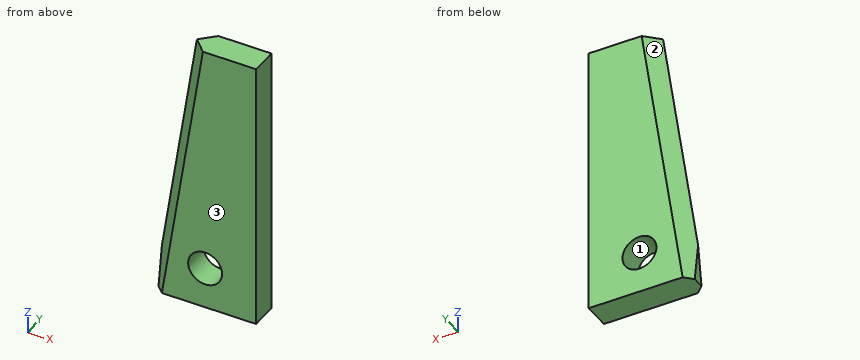
from build123d import *

# Parameters (mm, degrees)
F0_W     = 19.05
F0_H     = 50.8
F1_DEPTH = 5.08
F3_D     = 6.35
F5_DEPTH = 25.4
F6_SIZE  = 2.53999


# Not quite as in the source:
# - a fillet or chamfer is up to 0.001 mm smaller than in the source, because OpenCascade refuses the exact size


with BuildPart() as f1:
    # F0 (on Front) → F1 (new body)
    with BuildSketch(Plane.XZ):
        with Locations((-9.525, 25.4)):
            Rectangle(F0_W, F0_H)
    extrude(amount=F1_DEPTH)

    # F3 (through all)
    with Locations(Plane.XZ.offset(5.08)):
        with Locations((-9.525, 7.7354544774)):
            Hole(F3_D / 2)

    # F4 (on face) → F5 (cut)
    with BuildSketch(Plane.XZ.offset(5.08)):
        Polygon((-19.05, 7.4566449039), (-12.5023688375, 50.8), (-19.05, 50.8), align=None)
    extrude(amount=-F5_DEPTH, mode=Mode.SUBTRACT)

    # F6 (size 2.54 in the source; OpenCascade refuses exactly that, so slightly less here)
    f6_edges = [f1.edges().sort_by_distance(p)[0] for p in [
        (-15.776184, -5.08, 29.128322),
        (-15.776184, 0, 29.128322),
    ]]
    chamfer(f6_edges, length=F6_SIZE)


solid = f1.part
Read the model definition and answer for the solid it produces. Units are mm, in the model's axes. Face numbers are marked on the shaded views. Round coordinates to 2 decimals unless told otherwise and drop trailing zeros. Order: outer loops, then holes, each group sorted by start corner. A loop starts at its lowest first (then second) coordinate and runs counter-clockwise, first axis right, second up. Notation, with made-up numbers: (42, 56.25) - (99, 56.25) arc R21 cw to (99, 82.25) - close; hole circle Ø2 at (-10.5, -33). An arc over 180 degrees is marked (long way). Use one line per item in the form item = value. Start each with the question number.
(1) Find the intervals of material crossed by line 1 along X through (y, z) = (-2.75, 6.5); line 2 along X through (y, z) = (-3.75, 8); line 3 along Z through (x, y) = (-9.25, -3.5), in increasing order. Write a range as from..to.
(2) Flat-ended cylindrical pins translate along their axes: pin 1 Ø1.5 at (y, z) = (-1.5, 39) entering from -X; pin 2 Ø4 at (x, z) = (-15, 27) entering from +Y. Find the tip coordinate at first contact, or state that the pin passes through.
(3) Determine the mould class of the marked faces 1, 2 and 3 for opening direction X: +X half, -X half, draft (parallel to the pull), parting line (faces both ways), or undercut.
(4) The part is cut by section B-B (y = -3.05). Give the vertices of the cut face in (x, z) (3 decimals).
Checked values:
q1.line_1 = -18.98..-12.45, -6.6..0
q1.line_2 = -17.74..-12.69, -6.36..0
q1.line_3 = 0..4.57, 10.9..50.8
q2.pin_1 = -14
q2.pin_2 = 0
q3.face_1 = undercut
q3.face_2 = -X half
q3.face_3 = draft
q4.outline = (-19.05, 0) - (0, 0) - (0, 50.8) - (-11.987, 50.8) - (-19.05, 4.042) - close; hole circle Ø6.35 at (-9.525, 7.735)
